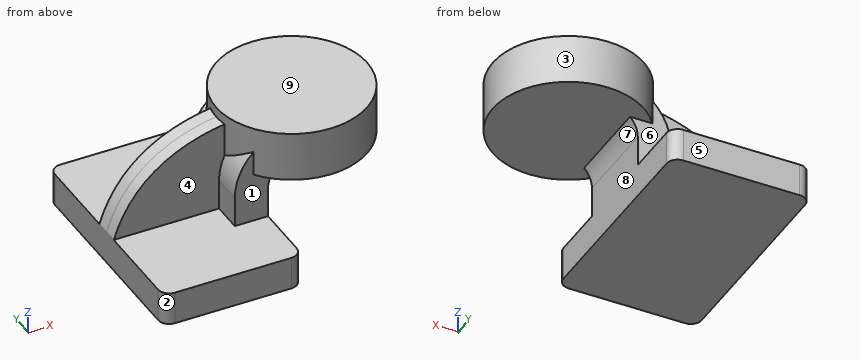
from build123d import *

# Parameters (mm, degrees)
F1_DEPTH = 63.5
F2_DEPTH = 25.4
F3_DEPTH = 7.9375
F0_W     = 43.2026712656
F0_H     = 28.575
F5_R     = 6.35


with BuildPart() as f1:
    # F0 (on Front) → F1 (new body, symmetric)
    with BuildSketch(Plane.XZ):
        Polygon((39.6875, -9.525), (39.6875, 9.525), (20.6375, 9.525), (-39.6875, 9.525), (-39.6875, -9.525), align=None)
    extrude(amount=F1_DEPTH, both=True)

    # F0 (on Front) → F2 (join, symmetric)
    with BuildSketch(Plane.XZ):
        with BuildLine():
            Line((20.6375, 9.525), (39.6875, 9.525))
            Line((39.6875, 9.525), (39.6875, 27.0256))
            ThreePointArc((39.6875, 27.0256), (44.3371798487, 38.2509201513), (55.5625, 42.9006))
            Line((55.5625, 42.9006), (58.7375, 42.9006))
            Line((58.7375, 42.9006), (58.7375, 61.9506))
            Line((58.7375, 61.9506), (55.5625, 61.9506))
            ThreePointArc((55.5625, 61.9506), (30.8667956671, 51.7213043329), (20.6375, 27.0256))
            Line((20.6375, 27.0256), (20.6375, 9.525))
        make_face()
        Polygon((58.7375, 66.675), (58.7375, 61.9506), (58.7375, 42.9006), (58.7375, 38.1), (66.3348287344, 38.1), (66.3348287344, 66.675), align=None)
    extrude(amount=F2_DEPTH, both=True)

    # F0 (on Front) → F3 (join, symmetric)
    with BuildSketch(Plane.XZ):
        with BuildLine():
            Line((-39.6875, 9.525), (20.6375, 9.525))
            Line((20.6375, 9.525), (20.6375, 27.0256))
            ThreePointArc((20.6375, 27.0256), (30.8667956671, 51.7213043329), (55.5625, 61.9506))
            Line((55.5625, 61.9506), (58.7375, 61.9506))
            add(Edge.make_bspline(
                [(-39.6875, 9.525), (-25.5478955805, 54.2332231998), (16.1354914308, 65.4384344816), (58.7375, 61.9506)],
                knots=[0, 0, 0, 0, 111.5164748383, 111.5164748383, 111.5164748383, 111.5164748383], degree=3))
        make_face()
    extrude(amount=F3_DEPTH, both=True)

    # F0 (on Front) → F4 (revolve)
    with BuildSketch(Plane.XZ):
        with Locations((87.9361643672, 52.3875)):
            Rectangle(F0_W, F0_H)
    revolve(axis=Axis((66.3348287344, 0, 52.3875), (0, 0, 1)))

    # F5
    f5_edges = [f1.edges().sort_by_distance(p)[0] for p in [
        (39.6875, -63.5, 0),
        (-39.6875, -63.5, 0),
        (39.6875, 63.5, 0),
        (-39.6875, 63.5, 0),
    ]]
    fillet(f5_edges, radius=F5_R)


solid = f1.part
Build history of the part. All positions in model axes, mm. Face numbers are marked on the shaded views. A direction names the side the tool comes from. Round coordinates to 2 decimals unless told otherwise and drop trailing zeros. Write each loop counter-clockwise with the first axis right and the second up, starting at its lowest first coordinate (ties: lowest second). Pieces come first, ordered by that corner, then holes. Notation, with made-up numbers: M 19.5,-18.5 L 56.5,-18.5 A24 cw 56.5,1.5 Z; hole C -1,4.5 d8. An arc over 180 degrees is marked long. Answer as a JSON object with one key per item and string values. Group by question number.
(1) Cut at C-C (x = 91.5). Give the cut face in (y, z) (3 decimals).
(2) Cut at B-B (y = -46). Give the cut face in (x, z) (1 decimal).
(3) Cut at A-A (z = -3.5). Give the cut face in (x, y).
(4) Flat gauge pins, fed straight in: pin 1 (8.5 mm diameter, centred on y = -17, z = 21, fed in from -X); pin 2 (8 mm diameter, centred on x = 9.5, z = 54.5, fed in from +Y); pin 3 (7 mm diameter, centred on x = 30.5, z = 27, fed in from -Y). Where does each tip first touch, or does it go through?
(5) Which spindle directions (+Z, -Z, +X, -X, +Y, -Y) get a long thin tool onto all of the face, cutting with end or side? Do the marked faces 1, 2, 3, 4 and 5. Say none if no direction does.
(6) Mould opens along Z. For the marked faces 6, 7, 8 and 9 say: pulls with the +Z half, pulls with the -Z half, needs draft (parallel to the pull), parting line crosses it, or undercut.
(7) Drill centre lines: L1, parallel to Z at x = -22, y = 54 (3 decimals); L2, parallel to Z at x = 65.5, y = -10 (3 decimals); L3, parallel to Y at x = 0.5, z = 42.5. Where is each one in solid material? Low to high.
Responses:
{
 "1": {"outline": "M -35.117,38.1 L 35.117,38.1 L 35.117,66.675 L -35.117,66.675 Z"},
 "2": {"outline": "M -39.7,-9.5 L 39.7,-9.5 L 39.7,9.5 L -39.7,9.5 Z"},
 "3": {"outline": "M -39.69,-57.15 A6.35 ccw -33.34,-63.5 L 33.34,-63.5 A6.35 ccw 39.69,-57.15 L 39.69,57.15 A6.35 ccw 33.34,63.5 L -33.34,63.5 A6.35 ccw -39.69,57.15 Z"},
 "4": {"pin 1": "stops at x = 20.64", "pin 2": "stops at y = 7.94", "pin 3": "stops at y = -25.4"},
 "5": {"face 1": "-X, -Y", "face 2": "+Z, -Z, -X, -Y", "face 3": "+Z", "face 4": "+Z, -X, -Y", "face 5": "+Z, -Z, +X, -X, +Y"},
 "6": {"face 6": "undercut", "face 7": "pulls with the -Z half", "face 8": "needs draft", "face 9": "pulls with the +Z half"},
 "7": {"L1": "z = -9.525 to 9.525", "L2": "z = 38.1 to 66.675", "L3": "y = -7.94 to 7.94"}
}
